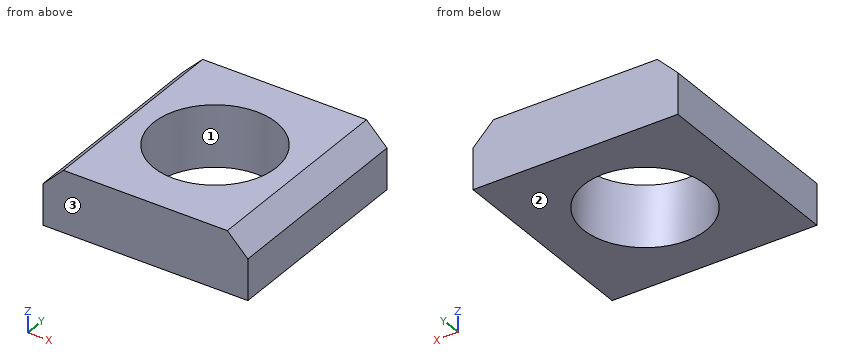
from build123d import *

# Parameters (mm, degrees)
SKETCH_W        = 10
SKETCH_H        = 10
SKETCH_R        = 3
PAD_DEPTH       = 3
CHAMFER_SIZE    = 1
CHAMFER001_SIZE = 1


with BuildPart() as part:
    # Sketch → Pad (new body)
    with BuildSketch(Plane.XY):
        with Locations((5, 5)):
            Rectangle(SKETCH_W, SKETCH_H)
        with Locations((5, 5)):
            Circle(SKETCH_R, mode=Mode.SUBTRACT)
    extrude(amount=PAD_DEPTH)

    # Chamfer
    chamfer_edges = [part.edges().sort_by_distance(p)[0] for p in [
        (0, 5, 3),
    ]]
    chamfer(chamfer_edges, length=CHAMFER_SIZE)

    # Chamfer001
    chamfer001_edges = [part.edges().sort_by_distance(p)[0] for p in [
        (10, 5, 3),
    ]]
    chamfer(chamfer001_edges, length=CHAMFER001_SIZE)


solid = part.part
Model file for the job. Use its own axes, mm. Face numbers are marked on the shaded views. Round coordinates to 2 decimals unless told otherwise and drop trailing zeros. Order: outer loops, then holes, each group sorted by start corner. A loop starts at its lowest first (then second) coordinate and runs counter-clockwise, first axis right, second up.
(1) Drill centre lines: line 1 (Y direction, x = 5, z = 0.65); line 2 (Y direction, x = 2.75, z = 2.4). Where is each one in solid material? Low to high.
(2) Band-saw the part on B-B (y = 5). List the corners of the cut face in (x, z).
(3) Band-saw the part on D-D (x = 3). List the corners of the cut face in (y, z).
(4) Pin check, flat tip, straight feed: pin 1 (5 mm diameter, centred on x = 5, y = 5, fed in from +Z). Stop position of the tip, or through.
(5) Band-saw the part on C-C (z = 0.55). List the corners of the cut face in (x, y), then the cut area to 3 significant figures.
(6) Band-saw the part on A-A (x = 5). List the corners of the cut face in (y, z), then the cut area to 3 significant figures.
(7) Pull direction Y, two halves, no side cores. Call the marked faces 1, 2 and 3: released by +Y, released by -Y, zero draft, split by the parting line, or undercut.
Verdict:
1. line 1: y = 0 to 2, 8 to 10
1. line 2: y = 0 to 3.02, 6.98 to 10
2. outline: (0, 0) - (2, 0) - (2, 3) - (1, 3) - (0, 2) - close; (8, 0) - (10, 0) - (10, 2) - (9, 3) - (8, 3) - close
3. outline: (0, 0) - (2.76, 0) - (2.76, 3) - (0, 3) - close; (7.24, 0) - (10, 0) - (10, 3) - (7.24, 3) - close
4. pin 1: passes through
5. outline: (0, 0) - (10, 0) - (10, 10) - (0, 10) - close; hole circle Ø6 at (5, 5)
5. area: 71.7 mm2
6. outline: (0, 0) - (2, 0) - (2, 3) - (0, 3) - close; (8, 0) - (10, 0) - (10, 3) - (8, 3) - close
6. area: 12.0 mm2
7. face 1: undercut
7. face 2: zero draft
7. face 3: released by -Y
